Study the drawing (mm; zero at the part's minimum x, y, z) and answer. A direction names the side the tool comes from. Coordinates: 2 decimals unless noted, no trailing zeros. Write each loop counter-clockwise with the first axis right and the second up, starting at its lowest first coordinate (ties: lowest second). Pieces come first, ordered by that corner, then holes. Notation, with made-up numbers: (14, 88) -> (67, 88) arc R23 ccw to (67, 102) -> close; hole circle Ø7 at (-13.5, 32). An arc over 180 degrees is marked (long way). Write item = value, one per line. Start each with the question number.
1) A tool of negligible diameter and unlimited length cuts with its end or side. For the marked faces 4, 5, 6, 7 and 8, from which of +Z, -Z, +X, -X, +Y, -Y can it reach the whole face along a straight path? Write none if from no direction.
2) Section A-A (z = 33.5) is taken. Determine the outline of the cut face in (x, y), plus the area to 3 significant figures.
3) Section D-D (y = 120) is taken. Determine the outline of the cut face in (x, z).
4) For a pull along X with two mould halves and no side action, classify the marked faces 1, 2 and 3 as released by +X, released by -X, zero draft, split by the parting line, or undercut.
5) Find the intervals of material crossed by line 1 along X through (y, z) = (21.5, 42); line 2 along Z through (x, y) = (66.5, 24.5); line 3 along X through (y, z) = (14, 58), in increasing order. Write a range as from..to.
6) Flat-ended cylindrical pins translate along their axes: pin 1 Ø8 at (x, y) = (77, 111) entering from -Z; pin 2 Ø4.5 at (x, z) = (115.5, 33.5) entering from +Y; pin 3 Ø2.5 at (x, z) = (116, 22.5) entering from -Y. Find the tip coordinate at first contact, or state that the pin passes through.
7) Section C-C (x = 117.5) is taken. Determine the outline of the cut face in (y, z), plus the area to 4 significant figures.
8) Section B-B (y = 15) is taken. Determine the outline of the cut face in (x, z), plus the area to 3 significant figures.
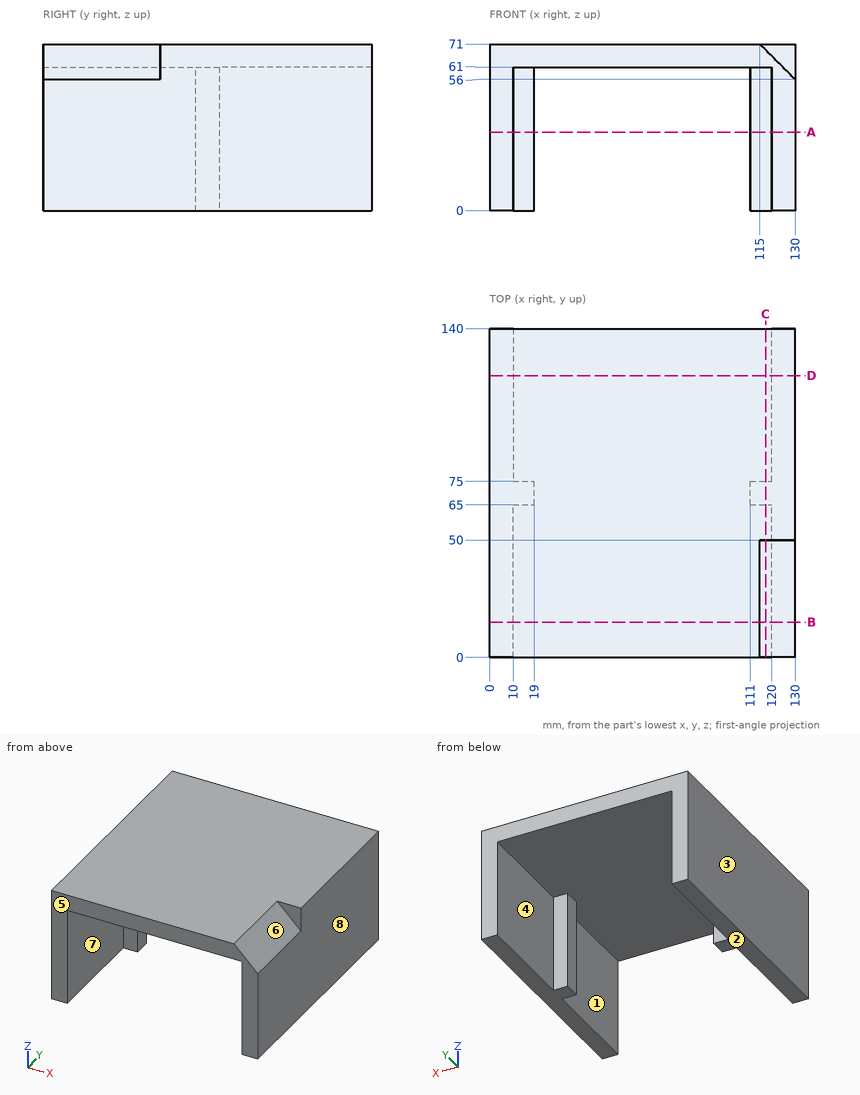
Answer key:
q1.face_4 = -Z, +Y
q1.face_5 = +Z, -Z, +X, -X, -Y
q1.face_6 = +Z, +X, -Y
q1.face_7 = -Z, -Y
q1.face_8 = +Z, -Z, +X, +Y, -Y
q2.outline = (0, 0) -> (10, 0) -> (10, 65) -> (19, 65) -> (19, 75) -> (10, 75) -> (10, 140) -> (0, 140) -> close; (111, 65) -> (120, 65) -> (120, 0) -> (130, 0) -> (130, 140) -> (120, 140) -> (120, 75) -> (111, 75) -> close
q2.area = 2,980 mm^2
q3.outline = (0, 0) -> (10, 0) -> (10, 61) -> (120, 61) -> (120, 0) -> (130, 0) -> (130, 71) -> (0, 71) -> close
q4.face_1 = undercut
q4.face_2 = zero draft
q4.face_3 = released by -X
q5.line_1 = 0..10, 120..130
q5.line_2 = 61..71
q5.line_3 = 0..10, 120..128
q6.pin_1 = 61
q6.pin_2 = 75
q6.pin_3 = 65
q7.outline = (0, 61) -> (65, 61) -> (65, 0) -> (75, 0) -> (75, 61) -> (140, 61) -> (140, 71) -> (50, 71) -> (50, 68.5) -> (0, 68.5) -> close
q7.area = 1,885 mm^2
q8.outline = (0, 0) -> (10, 0) -> (10, 61) -> (120, 61) -> (120, 0) -> (130, 0) -> (130, 56) -> (115, 71) -> (0, 71) -> close
q8.area = 2,410 mm^2
